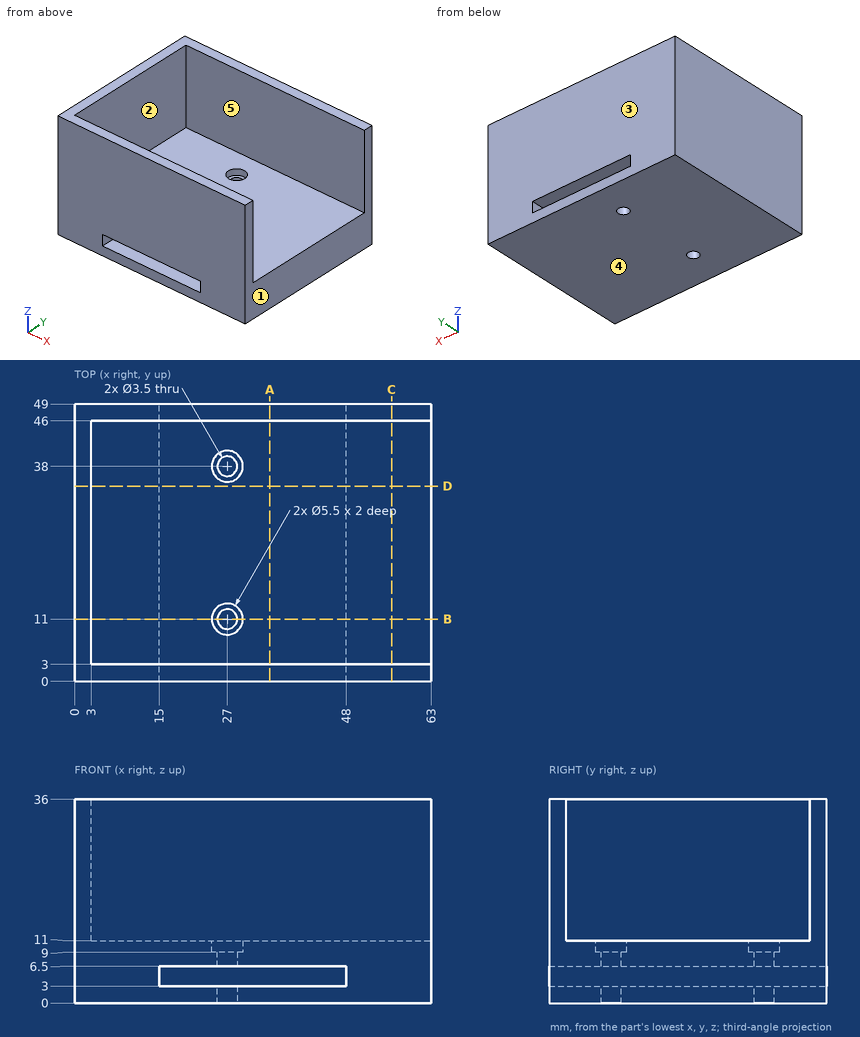
Check sheet for the drawn part. Datum: minimum x, y, z corner. Units: mm. A direction names the side the tool comes from. Round coordinates to 2 decimals unless told otherwise and drop trailing zeros. Order: outer loops, then holes, each group sorted by start corner. A loop starts at its lowest first (then second) coordinate and runs counter-clockwise, first axis right, second up. Notation, with made-up numbers: M -7.5,20 L 19.5,20 A38 ccw 19.5,59 Z; hole C 28,-35.5 d9. An arc over 180 degrees is marked long. Answer in a Markdown table with one row per item.
(1) Section check C-C on x = 56. Record the boundary of the cut face in (y, z), plus the area to 3 significant figures.
Findings:
| item | result |
|---|---|
| outline | M 0,0 L 49,0 L 49,36 L 46,36 L 46,11 L 3,11 L 3,36 L 0,36 Z |
| area | 689 mm^2 |
(2) Gauge pin test, flat ends, axial feed: pin 1 (1 mm diameter, centred on x = 38.5, y = 34.5, fed in from +Z); pin 2 (2 mm diameter, centred on x = 27, y = 38, fed in from -Z). Record the tip position at first contact, or that the pin passes through.
Findings:
| item | result |
|---|---|
| pin 1 | stops at z = 11 |
| pin 2 | passes through |
(3) Set-up check for the marked faces 4 and 5: record each of +Z, -Z, +X, -X, +Y, -Y from which the full face is reachable in a straight line by a thin tool's end or side.
Findings:
| item | result |
|---|---|
| face 4 | -Z, +X, -X, +Y, -Y |
| face 5 | +Z, +X |
(4) Section check D-D on y = 34.5. Record the boundary of the cut face in (x, z).
Findings:
| item | result |
|---|---|
| outline | M 0,0 L 63,0 L 63,11 L 3,11 L 3,36 L 0,36 Z; hole M 15,3 L 48,3 L 48,6.5 L 15,6.5 Z |
(5) Draft check along Y on the marked faces 1, 2 and 3. Enter one of: +Y half, -Y half, draft (parallel to the pull), parting line (faces both ways), or undercut.
Findings:
| item | result |
|---|---|
| face 1 | draft |
| face 2 | undercut |
| face 3 | +Y half |
(6) Section check A-A on x = 34.5. Record the boundary of the cut face in (y, z), plus the area to 4 significant figures.
Findings:
| item | result |
|---|---|
| outline | M 0,0 L 49,0 L 49,3 L 0,3 Z; M 0,6.5 L 49,6.5 L 49,36 L 46,36 L 46,11 L 3,11 L 3,36 L 0,36 Z |
| area | 517.5 mm^2 |
(7) Section check B-B on y = 11. Record the boundary of the cut face in (x, z).
Findings:
| item | result |
|---|---|
| outline | M 0,0 L 25.25,0 L 25.25,3 L 15,3 L 15,6.5 L 25.25,6.5 L 25.25,9 L 24.25,9 L 24.25,11 L 3,11 L 3,36 L 0,36 Z; M 28.75,0 L 63,0 L 63,11 L 29.75,11 L 29.75,9 L 28.75,9 L 28.75,6.5 L 48,6.5 L 48,3 L 28.75,3 Z |
(8) Material ranges on line 1 along Y through (x, z) = (27, 2); line 2 along Y through (x, z) = (29, 23.5); line 3 along X through (y, z) = (20.5, 4), recorded low to high. Write a range as from..to.
Findings:
| item | result |
|---|---|
| line 1 | y = 0..9.25, 12.75..36.25, 39.75..49 |
| line 2 | y = 0..3, 46..49 |
| line 3 | x = 0..15, 48..63 |
